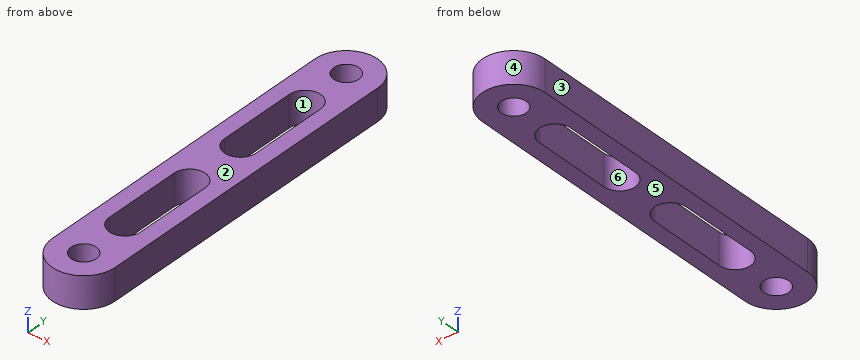
```python
from build123d import *

# Parameters (mm, degrees)
SKETCH1_R           = 4
BOSS_EXTRUDE1_DEPTH = 10


with BuildPart() as part:
    # Sketch1 → Boss-Extrude1 (new body)
    with BuildSketch(Plane.XY):
        with BuildLine():
            Line((-10, -50.8), (-10, 50.8))
            ThreePointArc((-10, 50.8), (0, 60.8), (10, 50.8))
            Line((10, 50.8), (10, -50.8))
            ThreePointArc((10, -50.8), (0, -60.8), (-10, -50.8))
        make_face()
        with Locations((0, -50.8)):
            Circle(SKETCH1_R, mode=Mode.SUBTRACT)
        with Locations((0, 50.8)):
            Circle(SKETCH1_R, mode=Mode.SUBTRACT)
        with BuildLine():
            Line((-5, -34.8), (-5, -9.8))
            ThreePointArc((-5, -9.8), (0, -4.8), (5, -9.8))
            Line((5, -9.8), (5, -34.8))
            ThreePointArc((5, -34.8), (0, -39.8), (-5, -34.8))
        make_face(mode=Mode.SUBTRACT)
        with BuildLine():
            Line((5, 34.8), (5, 9.8))
            ThreePointArc((5, 9.8), (0, 4.8), (-5, 9.8))
            Line((-5, 9.8), (-5, 34.8))
            ThreePointArc((-5, 34.8), (0, 39.8), (5, 34.8))
        make_face(mode=Mode.SUBTRACT)
    extrude(amount=BOSS_EXTRUDE1_DEPTH)


solid = part.part
```
For this review, take the finished solid that the model builds, in its own axes (mm). Face numbers are marked on the shaded views. A direction names the side the tool comes from. Coordinates: 2 decimals unless noted, no trailing zeros. Loops run counter-clockwise (first coordinate to the right, second up) from the corner with the lowest first, then second, coordinate; pieces in that order, holes last.
1. Mouldability with a two-part tool opening along X and no side actions: class the marked faces 1, 2, 3 and 4 as +X half, -X half, draft (parallel to the pull), parting line (faces both ways), or undercut.
2. For the marked faces 5 and 6, list the 3-axis set-ups (+Z, -Z, +X, -X, +Y, -Y) from which the entire face can be reached by the end or side of a thin tool; tool diameter is ignored.
3. Insertion check: P1, Ø3, axis at x = -6.5, z = 4, coming from the +Y side; P2, Ø6, axis at x = 4.5, z = 2, coming from the +Y side. Each pin has a flat end and moves straight along its axis. Give the tip position at first contact, or say it passes through.
4. Add section B-B, the plane x = 0. Give the boundary of the cut face in (y, z).
5. Add section C-C, the plane x = 7. Give the boundary of the cut face in (y, z), then the cut area to 3 significant figures.
6. For line 1 (Y direction, x = 0, z = 6.5); line 2 (Y direction, x = 1.5, z = 8.25); line 3 (X direction, y = -10.5, z = 4.75), list the stretches that pass through material, from the lowest coordinate up.
7. Add section A-A, the plane z = 6. Give the boundary of the cut face in (x, y), then the cut area to 3 significant figures.
Result:
1. face 1: undercut
1. face 2: draft
1. face 3: -X half
1. face 4: parting line
2. face 5: -Z, +X, -X, +Y, -Y
2. face 6: +Z, -Z
3. P1: stops at y = 59.46
3. P2: stops at y = 60.69
4. outline: (-60.8, 0) - (-54.8, 0) - (-54.8, 10) - (-60.8, 10) - close; (-46.8, 0) - (-39.8, 0) - (-39.8, 10) - (-46.8, 10) - close; (-4.8, 0) - (4.8, 0) - (4.8, 10) - (-4.8, 10) - close; (39.8, 0) - (46.8, 0) - (46.8, 10) - (39.8, 10) - close; (54.8, 0) - (60.8, 0) - (60.8, 10) - (54.8, 10) - close
5. outline: (-57.94, 0) - (57.94, 0) - (57.94, 10) - (-57.94, 10) - close
5. area: 1,160 mm2
6. line 1: y = -60.8 to -54.8, -46.8 to -39.8, -4.8 to 4.8, 39.8 to 46.8, 54.8 to 60.8
6. line 2: y = -60.69 to -54.51, -47.09 to -39.57, -5.03 to 5.03, 39.57 to 47.09, 54.51 to 60.69
6. line 3: x = -10 to -5, 5 to 10
7. outline: (-10, -50.8) arc R10 ccw to (10, -50.8) - (10, 50.8) arc R10 ccw to (-10, 50.8) - close; hole (-5, -34.8) arc R5 ccw to (5, -34.8) - (5, -9.8) arc R5 ccw to (-5, -9.8) - close; hole (-5, 9.8) arc R5 ccw to (5, 9.8) - (5, 34.8) arc R5 ccw to (-5, 34.8) - close; hole circle Ø8 at (0, -50.8); hole circle Ø8 at (0, 50.8)
7. area: 1,590 mm2
